Read the model definition and answer for the solid it produces. Units are mm, in the model's axes. A direction names the side the tool comes from. Round coordinates to 2 decimals unless told otherwise and drop trailing zeros. Write each loop counter-clockwise with the first axis right and the second up, starting at its lowest first coordinate (ties: lowest second). Pieces come first, ordered by that corner, then holes. Notation, with made-up numbers: (-15, -14.75) - (39, -14.75) arc R26 cw to (39, 20.25) - close; hole circle Ø6 at (29, -27). An arc over 180 degrees is marked (long way). One line per item, written item: value. Start each with the question number.
(1) A cutting plane is placed at A-A, the plane z = -82. Determine the outline of the cut face in (x, y).
(2) Flat-ended cylindrical pins translate along their axes: pin 1 Ø4 at (x, y) = (7.51, 28.01) entering from -Z; pin 2 Ø4.5 at (y, z) = (0, -82) entering from +X; pin 3 Ø1.5 at (y, z) = (-10.5, -8) entering from -X. Find the tip coordinate at first contact, or state that the pin passes through.
(3) A cutting plane is placed at B-B, the plane z = 1.5. State how many separate pieces and enclosed holes the cut face has, plus the area to 3 significant figures.
(4) The mould has two halves that part along Y. Classify faces 5 (the face through (-29.536, -8.138, 2.745)), 6 (the face through (0.07, -23.49, -80.35)), 7 (the face through (-23.977, -1.055, -37.336)): +Y half, -Y half, draft (parallel to the pull), parting line (faces both ways), or undercut.
(5) For faces 1 (the face through (-23.49, -0.07, -80.35)), 2 (the face through (-26.07, 0.65, 7.75)), 3 (the face through (-17.612, 17.743, 2.93)), 4 (the face through (23.846, -7.509, -6.084)), determine the directions among +Z, -Z, +X, -X, +Y, -Y from which every point of the face is accessible in a straight line to the end or side of a thin tool.
(6) Find the intervals of material crossed by L1, parallel to Y at x = 0, z = 2.75; L2, parallel to Z at x = -22, y = -28; L3, parallel to Y at x = 15, z = -1.5, in increasing order.
from build123d import *
from build123d.topology import SkipClean

# Parameters (mm, degrees)
EXTRUDE_START                = 8
SKETCH_5_R                   = 35
SKETCH_5_R_2                 = 22
EXTRUDE_1_DEPTH              = 8
SKETCH_9_W                   = 1.65
SKETCH_9_H                   = 37.5
SKETCH_2_R                   = 1.5
CUT_EXTRUDE_1_DEPTH          = 110.674519
PATTERN_CIRCULAR_1_COUNT     = 4
HOLE_WIZARD_M4_4_D           = 3.3
HOLE_WIZARD_M4_4_CSINK_D     = 4.05
HOLE_WIZARD_M4_4_CSINK_ANGLE = 90
HOLE_WIZARD_1_AT_2_COUNT     = 2
HOLE_WIZARD_1_AT_2_PITCH     = 41.012193
HOLE_WIZARD_1_AT_3_COUNT     = 2
HOLE_WIZARD_1_AT_3_PITCH     = 58
HOLE_WIZARD_1_AT_4_COUNT     = 2
HOLE_WIZARD_1_AT_4_PITCH     = 41.012193
CHAMFER_1_SIZE               = 2
CHAMFER_2_SIZE               = 1


# Some blends are built 0.0001 mm under size
with BuildPart() as part:
    # 草图1 → 旋转1 (revolve)
    with BuildSketch(Plane(origin=(0, 0, 0), x_dir=(1, 0, 0), z_dir=(0, 1, 0))):
        Polygon((37.5, 0), (37.5, 2), (25, 2), (25, 12), (24, 12), (24, 62), (25, 62), (25, 98), (22, 98), (22, 0), align=None)
    revolve(axis=Axis((0, 0, 0), (0, 0, -1)))

    # 草图5 → 凸台-拉伸1 (add)
    with BuildSketch(Plane.XY.offset(EXTRUDE_START)):
        Circle(SKETCH_5_R)
        Circle(SKETCH_5_R_2, mode=Mode.SUBTRACT)
    extrude(amount=-EXTRUDE_1_DEPTH)

    # 草图9 → M4 螺纹孔2 (revolve, cut)
    with BuildSketch(Plane(origin=(0, 0, -82), x_dir=(0, 0, -1), z_dir=(1, 0, 0))):
        with Locations((0.825, 18.75)):
            Rectangle(SKETCH_9_W, SKETCH_9_H)
    hole_wizard_m4_2 = revolve(axis=Axis((0, -6.35, -82), (0, 1, 0)), mode=Mode.SUBTRACT)

    # 草图2 → 切除-拉伸1 (cut, through all)
    with SkipClean():  # the faces are left unmerged after this step: merging them gives an invalid solid
        with BuildSketch(Plane(origin=(0, 0, -2), x_dir=(-1, 0, 0), z_dir=(0, 0, -1))):
            with Locations((0, 29)):
                Circle(SKETCH_2_R)
            with Locations((29, 0)):
                Circle(SKETCH_2_R)
            with Locations((0, -29)):
                Circle(SKETCH_2_R)
            with Locations((-29, 0)):
                Circle(SKETCH_2_R)
            with BuildLine():
                ThreePointArc((26.846788, 15.5), (21.92031, 21.92031), (15.5, 26.846788))
                ThreePointArc((15.5, 26.846788), (11.401924, 25.748711), (12.5, 21.650635))
                ThreePointArc((12.5, 21.650635), (17.67767, 17.67767), (21.650635, 12.5))
                ThreePointArc((21.650635, 12.5), (25.748711, 11.401924), (26.846788, 15.5))
            make_face()
            with BuildLine():
                ThreePointArc((-26.846788, -15.5), (-21.92031, -21.92031), (-15.5, -26.846788))
                ThreePointArc((-15.5, -26.846788), (-11.401924, -25.748711), (-12.5, -21.650635))
                ThreePointArc((-12.5, -21.650635), (-17.67767, -17.67767), (-21.650635, -12.5))
                ThreePointArc((-21.650635, -12.5), (-25.748711, -11.401924), (-26.846788, -15.5))
            make_face()
        extrude(amount=-CUT_EXTRUDE_1_DEPTH, mode=Mode.SUBTRACT)

    # 阵列(圆周)1: M4 螺纹孔2 ×4 about axis
    with SkipClean():  # the faces are left unmerged after this step: merging them gives an invalid solid
        pattern_circular_1_axis = Axis((0, 0, 0), (0, 0, -1))
        for i in range(1, PATTERN_CIRCULAR_1_COUNT):
            add(hole_wizard_m4_2.rotate(pattern_circular_1_axis, i * 360 / PATTERN_CIRCULAR_1_COUNT), mode=Mode.SUBTRACT)

    # M4 螺纹孔4 (through all)
    with Locations(Plane.XY.offset(8)):
        with Locations((7.505752, 28.011849), (28.011849, 7.505752), (-7.505752, -28.011849), (-28.011849, -7.505752)):
            CounterSinkHole(HOLE_WIZARD_M4_4_D / 2, HOLE_WIZARD_M4_4_CSINK_D / 2, counter_sink_angle=HOLE_WIZARD_M4_4_CSINK_ANGLE)

    # 草图15 → 孔1 (revolve, cut)
    with SkipClean():  # the faces are left unmerged after this step: merging them gives an invalid solid
        with BuildSketch(Plane(origin=(-29, 0, 8), x_dir=(0, -1, 0), z_dir=(1, 0, 0))):
            Polygon((0, 0), (0, 106), (1.5, 106), (1.5, 2), (3, 0.5), (3, 0), align=None)
        hole_wizard_1 = revolve(axis=Axis((-29, 0, 14.130024), (0, 0, -1)), mode=Mode.SUBTRACT)

    # 孔1 at 2: 孔1 ×2
    with SkipClean():  # the faces are left unmerged after this step: merging them gives an invalid solid
        with Locations(*[Vector(0.7071067811865532, -0.7071067811865418, 0) * (i * HOLE_WIZARD_1_AT_2_PITCH) for i in range(1, HOLE_WIZARD_1_AT_2_COUNT)]):
            add(hole_wizard_1, mode=Mode.SUBTRACT)

    # 孔1 at 3: 孔1 ×2
    with SkipClean():  # the faces are left unmerged after this step: merging them gives an invalid solid
        with Locations(*[(i * HOLE_WIZARD_1_AT_3_PITCH, 0, 0) for i in range(1, HOLE_WIZARD_1_AT_3_COUNT)]):
            add(hole_wizard_1, mode=Mode.SUBTRACT)

    # 孔1 at 4: 孔1 ×2
    with SkipClean():  # the faces are left unmerged after this step: merging them gives an invalid solid
        with Locations(*[Vector(0.7071067811865457, 0.7071067811865495, 0) * (i * HOLE_WIZARD_1_AT_4_PITCH) for i in range(1, HOLE_WIZARD_1_AT_4_COUNT)]):
            add(hole_wizard_1, mode=Mode.SUBTRACT)

    # 倒角1
    # the kernel refuses this chamfer: 2 mm, written as the material it takes off along each edge
    with BuildSketch(Plane(origin=(24.248711, -14, -2), x_dir=(-0.3683025891242999, -0.9297059765562106, 0), z_dir=(0.9297059765562106, -0.3683025891242999, 0))) as chamfer_1_piece_1_section:
        Polygon((3 + CHAMFER_1_SIZE, 0), (3, -CHAMFER_1_SIZE), (3, 0), align=None)
    chamfer_1_piece_1 = revolve(axis=Axis((24.248711, -14, -2), (0, 0, -1)), revolution_arc=278.389028, mode=Mode.PRIVATE)
    chamfer_1_piece_1 = chamfer_1_piece_1 - Plane(origin=(0, 0, -1.316198), x_dir=(1, 0, 0), z_dir=(0, 0, -1)) * Cylinder(25, 21, mode=Mode.PRIVATE)
    add(chamfer_1_piece_1, mode=Mode.SUBTRACT)
    with BuildSketch(Plane(origin=(0, 0, -2), x_dir=(0.866025403784439, -0.49999999999999944, 0), z_dir=(0.49999999999999944, 0.866025403784439, 0))) as chamfer_1_piece_2:
        Polygon((31 + CHAMFER_1_SIZE, 0), (31, -CHAMFER_1_SIZE), (31, 0), align=None)
    revolve(axis=Axis((0, 0, -2), (0, 0, -1)), revolution_arc=30, mode=Mode.SUBTRACT)
    with BuildSketch(Plane(origin=(14, -24.248711, -2), x_dir=(0.5, -0.8660254037844387, 0), z_dir=(0.8660254037844387, 0.5, 0))) as chamfer_1_piece_3_section:
        Polygon((3 + CHAMFER_1_SIZE, 0), (3, -CHAMFER_1_SIZE), (3, 0), align=None)
    chamfer_1_piece_3 = revolve(axis=Axis((14, -24.248711, -2), (0, 0, -1)), revolution_arc=278.389028, mode=Mode.PRIVATE)
    chamfer_1_piece_3 = chamfer_1_piece_3 - Plane(origin=(0, 0, -1.445844), x_dir=(1, 0, 0), z_dir=(0, 0, -1)) * Cylinder(25, 21, mode=Mode.PRIVATE)
    add(chamfer_1_piece_3, mode=Mode.SUBTRACT)
    with BuildSketch(Plane(origin=(-24.248711, 14, -2), x_dir=(0.368302589124304, 0.9297059765562089, 0), z_dir=(-0.9297059765562089, 0.368302589124304, 0))) as chamfer_1_piece_4_section:
        Polygon((3 + CHAMFER_1_SIZE, 0), (3, -CHAMFER_1_SIZE), (3, 0), align=None)
    chamfer_1_piece_4 = revolve(axis=Axis((-24.248711, 14, -2), (0, 0, -1)), revolution_arc=278.389028, mode=Mode.PRIVATE)
    chamfer_1_piece_4 = chamfer_1_piece_4 - Plane(origin=(0, 0, -1.316197), x_dir=(1, 0, 0), z_dir=(0, 0, -1)) * Cylinder(25, 21, mode=Mode.PRIVATE)
    add(chamfer_1_piece_4, mode=Mode.SUBTRACT)
    with BuildSketch(Plane(origin=(0, 0, -2), x_dir=(-0.8660254037844394, 0.4999999999999989, 0), z_dir=(-0.4999999999999989, -0.8660254037844394, 0))) as chamfer_1_piece_5:
        Polygon((31 + CHAMFER_1_SIZE, 0), (31, -CHAMFER_1_SIZE), (31, 0), align=None)
    revolve(axis=Axis((0, 0, -2), (0, 0, -1)), revolution_arc=30, mode=Mode.SUBTRACT)
    with BuildSketch(Plane(origin=(-14, 24.248711, -2), x_dir=(-0.5000000000000014, 0.8660254037844378, 0), z_dir=(-0.8660254037844378, -0.5000000000000014, 0))) as chamfer_1_piece_6_section:
        Polygon((3 + CHAMFER_1_SIZE, 0), (3, -CHAMFER_1_SIZE), (3, 0), align=None)
    chamfer_1_piece_6 = revolve(axis=Axis((-14, 24.248711, -2), (0, 0, -1)), revolution_arc=278.389028, mode=Mode.PRIVATE)
    chamfer_1_piece_6 = chamfer_1_piece_6 - Plane(origin=(0, 0, -1.445844), x_dir=(1, 0, 0), z_dir=(0, 0, -1)) * Cylinder(25, 20, mode=Mode.PRIVATE)
    add(chamfer_1_piece_6, mode=Mode.SUBTRACT)

    # 倒角2
    chamfer_2_edges = [part.edges().sort_by_distance(p)[0] for p in [
        (-24, 0, -62),
        (-24, 0, -12),
    ]]
    chamfer(chamfer_2_edges, length=CHAMFER_2_SIZE - 0.0001)  # a hair under: the kernel refuses the full size


solid = part.part
Here are the results:
1. outline: (-24.95, -1.65) arc R25 ccw to (-1.65, -24.95) - (-1.65, -21.94) arc R22 cw to (-21.94, -1.65) - close; (-24.95, 1.65) - (-21.94, 1.65) arc R22 cw to (-1.65, 21.94) - (-1.65, 24.95) arc R25 ccw to start; (1.65, -24.95) arc R25 ccw to (24.95, -1.65) - (21.94, -1.65) arc R22 cw to (1.65, -21.94) - close; (1.65, 21.94) arc R22 cw to (21.94, 1.65) - (24.95, 1.65) arc R25 ccw to (1.65, 24.95) - close
2. pin 1: z = -2
2. pin 2: x = 25
2. pin 3: x = -23.02
3. separate pieces: 1
3. enclosed holes: 11
3. area: 2,030 mm²
4. face 5: undercut
4. face 6: draft
4. face 7: parting line
5. face 1: +X, -X
5. face 2: +Z
5. face 3: +Z, -Z
5. face 4: -Z
6. L1: -35 to -30.5, -27.5 to -22, 22 to 27.5, 30.5 to 35
6. L2: -2 to 0
6. L3: -34.37 to -28.64, -20 to -16.09, 16.09 to 34.37
